from build123d import *

# Parameters (mm, degrees)
F0_R     = 19.05
F1_DEPTH = 2.54
F3_R     = 1.041647
F3_R_2   = 1.054587
F3_R_3   = 1.562468
F3_R_4   = 0.960349
F3_R_5   = 1.983236
F3_R_6   = 1.104833
F3_R_7   = 1.99006
F3_R_8   = 1.983233
F3_R_9   = 1.622095
F4_DEPTH = 25.4
F6_R     = 0.702637
F7_DEPTH = 2.54
F8_R     = 1.5875
F9_DEPTH = 3.175


with BuildPart() as f1:
    # F0 (on Front) → F1 (new body)
    with BuildSketch(Plane.XZ):
        with Locations((-40.385999, 44.069)):
            Circle(F0_R)
    extrude(amount=-F1_DEPTH)

    # F3 (on face) → F4 (cut)
    with BuildSketch(Plane.XZ):
        with Locations((-40.877204, 56.347888)):
            Circle(F3_R)
        with Locations((-33.301067, 53.548012)):
            Circle(F3_R_2)
        with Locations((-29.348301, 47.618862)):
            Circle(F3_R_3)
        with Locations((-28.689506, 43.007299)):
            Circle(F3_R_4)
        with Locations((-31.98348, 35.760563)):
            Circle(F3_R_5)
        with Locations((-40.877204, 34.278274)):
            Circle(F3_R_6)
        with Locations((-48.947435, 35.760563)):
            Circle(F3_R_7)
        with Locations((-52.406106, 44.818986)):
            Circle(F3_R_8)
        with Locations((-47.794547, 53.548012)):
            Circle(F3_R_9)
    extrude(amount=-F4_DEPTH, mode=Mode.SUBTRACT)

    # F6 (on face) → F7 (join)
    with BuildSketch(Plane.XZ):
        with Locations((-40.731799, 44.465709)):
            Circle(F6_R)
    extrude(amount=F7_DEPTH)

    # F8 (on face) → F9 (join)
    with BuildSketch(Plane(origin=(0, 2.54, 0), x_dir=(-1, 0, 0), z_dir=(0, 1, 0))):
        with Locations((40.671818, 44.492617)):
            Circle(F8_R)
    extrude(amount=F9_DEPTH)


solid = f1.part
Read the model definition and answer for the solid it produces. Units are mm, in the model's axes. A direction names the side the tool comes from. Round coordinates to 2 decimals unless told otherwise and drop trailing zeros. Write each loop counter-clockwise with the first axis right and the second up, starting at its lowest first coordinate (ties: lowest second). Pieces come first, ordered by that corner, then holes.
1. The part is cut by section B-B, the plane x = -51.5. Determine the outline of the cut face in (y, z).
2. Given pin 1 Ø3 at (x, y) = (-40.5, -0.5) entering from -Z; pin 2 Ø5 at (x, z) = (-29.35, 47.62) entering from -Y; pin 3 Ø1 at (y, z) = (-1.5, 39.5) entering from +X; pin 4 Ø5 at (x, z) = (-48.95, 35.76) entering from +Y, each flat-ended and moving along its own axis, determine where each tip first touches the part or whether it passes through.
3. Determine the mould class of faces 1 (the face through (-49.08, 1.25, 52.56)), 2 (the face through (-41, 5.715, 45)), 3 (the face through (-40.328, 4.105, 42.943)) for opening direction X: pulls with the +X half, pulls with the -X half, needs draft (parallel to the pull), parting line crosses it, or undercut.
4. Straight lines are drawn through the part: L1, parallel to Z at x = -41.5, y = 1.5; L2, parallel to X at y = 0.75, z = 54; L3, parallel to Z at x = -29, y = 1.5. For each, find the intervals that lie inside material, in ascending order.
5. The part is cut by section C-C, the plane z = 38.5. Determine the outline of the cut face in (x, y).
6. The part is cut by section A-A, the plane y = 1. State how many separate pieces and enclosed holes the cut face has, then the cut area to 3 significant figures.
7. Which of the six approach directions +Z, -Z, +X, -X, +Y, -Y give full straight-line access (tool end or side, diameter ignored) to faces 4 (the face through (-40.062, -1.252, 44.677)), 5 (the face through (-31.596, 1.252, 27.168))?
8. The part is cut by section D-D, the plane x = -45. Determine the outline of the cut face in (y, z).
Values:
1. outline: (0, 28.6) - (2.54, 28.6) - (2.54, 43.05) - (0, 43.05) - close; (0, 46.58) - (2.54, 46.58) - (2.54, 59.54) - (0, 59.54) - close
2. pin 1: stops at z = 25.02
2. pin 2: stops at y = 0
2. pin 3: passes through
2. pin 4: stops at y = 2.54
3. face 1: undercut
3. face 2: needs draft
3. face 3: parting line crosses it
4. L1: z = 25.05 to 33.37, 35.19 to 55.51, 57.18 to 63.09
4. L2: x = -56.64 to -49.35, -46.24 to -34.25, -32.35 to -24.13
4. L3: z = 28.8 to 42.1, 43.92 to 46.1, 49.14 to 59.34
5. outline: (-58.6, 0) - (-22.17, 0) - (-22.17, 2.54) - (-58.6, 2.54) - close
6. separate pieces: 1
6. enclosed holes: 9
6. area: 1,070 mm2
7. face 4: -Y
7. face 5: +Y, -Y
8. outline: (0, 25.59) - (2.54, 25.59) - (2.54, 62.55) - (0, 62.55) - close
